Check sheet for the drawn part. Datum: minimum x, y, z corner. Units: mm. A direction names the side the tool comes from. Round coordinates to 2 decimals unless told otherwise and drop trailing zeros. Order: outer loops, then holes, each group sorted by start corner. A loop starts at its lowest first (then second) coordinate and runs counter-clockwise, first axis right, second up. Notation, with made-up numbers: (27.25, 6.5) -> (53.25, 6.5) arc R25 cw to (53.25, 25.5) -> close; hole circle Ø8 at (13.5, -32). An arc over 180 degrees is marked (long way). Use CSV: the item, a comma, the result in double quotes.
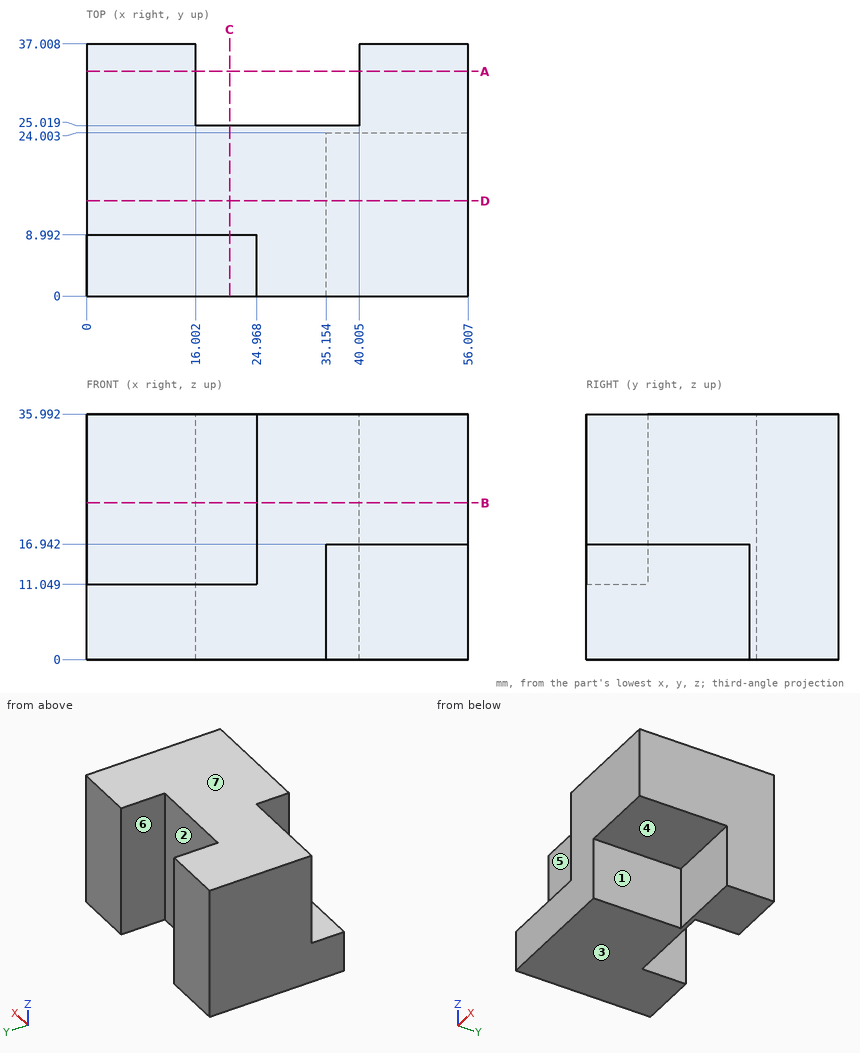
Q1. Sectioned sample at D-D, the plane y = 14. Enter the section's corners in (x, z), then the cut area to 3 significant figures.
Result sheet:
outline,"(0, 0) -> (35.15, 0) -> (35.15, 16.94) -> (56.01, 16.94) -> (56.01, 35.99) -> (0, 35.99) -> close"
area,"1,660 mm^2"
Q2. Sectioned sample at C-C, the plane x = 21. Enter the section's corners in (y, z), then the cut area to 3 significant figures.
Result sheet:
outline,"(0, 0) -> (25.02, 0) -> (25.02, 35.99) -> (8.99, 35.99) -> (8.99, 11.05) -> (0, 11.05) -> close"
area,"676 mm^2"
Q3. Sectioned sample at A-A, the plane y = 33. Enter the section's corners in (x, z) (1 decimal).
Result sheet:
outline,"(0, 0) -> (16, 0) -> (16, 36) -> (0, 36) -> close; (40, 0) -> (56, 0) -> (56, 36) -> (40, 36) -> close"
Q4. Mould release check, pull along X, two halves, no side actions. Record for the marked faces 1, 2 and 3: pulls with the +X half, pulls with the -X half, needs draft (parallel to the pull), parting line crosses it, or undercut.
Result sheet:
face 1,"pulls with the +X half"
face 2,"undercut"
face 3,"needs draft"
Q5. Go/stop test with flat-tipped pins: pin 1 (2 mm diameter, centred on x = 24.5, z = 13.5, fed in from +Y); pin 2 (18.5 mm diameter, centred on y = 12, z = 4.5, fed in from +X); pin 3 (6 mm diameter, centred on x = 40, z = 13.5, fed in from -Y). Record where each tip stops, or that it passes through.
Result sheet:
pin 1,"stops at y = 25.02"
pin 2,"stops at x = 35.15"
pin 3,"stops at y = 24"
Q6. Sectioned sample at B-B, the plane z = 23. Enter the section's corners in (x, y) (1 decimal), then the cut area to 3 significant figures.
Result sheet:
outline,"(0, 9) -> (25, 9) -> (25, 0) -> (56, 0) -> (56, 37) -> (40, 37) -> (40, 25) -> (16, 25) -> (16, 37) -> (0, 37) -> close"
area,"1,560 mm^2"
Q7. Access from +Z, -Z, +X, -X, +Y, -Y to the whole of each face (thin tool, end or side, straight path). Record for the marked faces 4, 5, 6 and 7.
Result sheet:
face 4,"-Z, +X, -Y"
face 5,"+Z, -X, -Y"
face 6,"+Z, -Z, +Y"
face 7,"+Z, +X, -X, +Y, -Y"
Q8. Scan lines: L1, parallel to X at y = 17, z = 3.5; L2, parallel to Y at x = 42.5, z = 4; L3, parallel to Z at x = 51.5, y = 19. Record each from-to range of solid material in increasing order.
Result sheet:
L1,"x = 0 to 35.15"
L2,"y = 24 to 37.01"
L3,"z = 16.94 to 35.99"
